Geometry check sheet. Reference: the model listing, model coordinates, mm. Coordinates: 2 decimals unless noted, no trailing zeros. Loops run counter-clockwise (first coordinate to the right, second up) from the corner with the lowest first, then second, coordinate; pieces in that order, holes last. Notation, with made-up numbers: (61.25, 71) -> (82.25, 71) arc R24 ccw to (82.25, 107) -> close; hole circle Ø8 at (39.5, -25.75). An arc over 180 degrees is marked (long way). Answer as a JSON object with one key per item and string values.
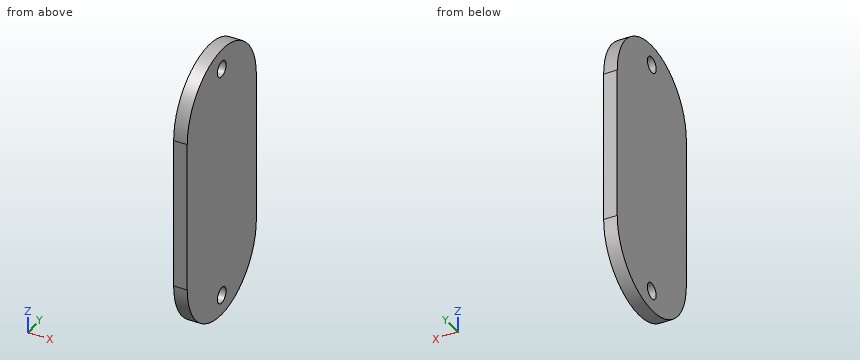
Autodesk Inventor part; units mm, degrees
ref_plane "YZ Plane" through (0, 0, 0) normal (1, 0, 0) x (0, 1, 0)
ref_plane "XZ Plane" through (0, 0, 0) normal (0, 1, 0) x (-1, 0, 0)
ref_plane "XY Plane" through (0, 0, 0) normal (0, 0, 1) x (1, 0, 0)
sketch "Sketch1" plane through (0, 0, 0) normal (1, 0, 0) x (0, 1, 0)
  arc A0 (-27.0381, 32.6694) -> (2.4619, 32.6694) centre (-12.2881, 32.6694) ccw
  arc A1 (-27.0381, 32.6694) -> (2.4619, 32.6694) centre (-12.2881, 32.6694) ccw
  arc A2 (-27.0381, 32.6694) -> (2.4619, 32.6694) centre (-12.2881, 32.6694) ccw
  line L0 (-27.0381, 32.6694) -> (-27.0381, 50.6694)
  line L1 (2.4619, 32.6694) -> (2.4619, 50.6694)
  line L2 (-27.0381, 50.6694) -> (-37.7302, 50.6694)
  arc A3 (2.4619, 68.6694) -> (-27.0381, 68.6694) centre (-12.2881, 68.6694) ccw
  arc A4 (2.4619, 68.6694) -> (-27.0381, 68.6694) centre (-12.2881, 68.6694) ccw
  arc A5 (2.4619, 68.6694) -> (-27.0381, 68.6694) centre (-12.2881, 68.6694) ccw
  line L3 (-27.0381, 68.6694) -> (-27.0381, 50.6694)
  line L4 (2.4619, 68.6694) -> (2.4619, 50.6694)
  circle A6 centre (-12.2881, 22.6694) radius 1.875
  circle A7 centre (-12.2881, 78.6694) radius 1.875
  point P0 (0, 0)
  dimension "d7" = 29.5
  dimension "d8" = 29.5
  dimension "d9" = 29.5
  dimension "d12" = 18
  dimension "d13" = 18
  dimension "d14" = 3.75
  dimension "d16" = 3.75
  dimension "d17" = 56
extrude "Extrusion1" add sketch "Sketch1" along normal blind 3.175
properties part number "clamp"
1. Section check B-B, the plane z = 22. Record the boundary of the cut face in (x, y) (3 decimals), then the cut area to 3 significant figures.
Evaluation:
{"outline": "(0, -22.473) -> (3.175, -22.473) -> (3.175, -14.04) -> (0, -14.04) -> close; (0, -10.537) -> (3.175, -10.537) -> (3.175, -2.103) -> (0, -2.103) -> close", "area": "53.6 mm^2"}
2. Section check D-D, the plane y = -24.25. Record the boundary of the cut face in (x, z) (3 decimals), then the cut area to 3 significant figures.
Evaluation:
{"outline": "(0, 24.039) -> (3.175, 24.039) -> (3.175, 77.299) -> (0, 77.299) -> close", "area": "169 mm^2"}
3. Thickness scan on probe 1 along Z at (x, y) = (0.5, -13.25); probe 2 along Y at (x, z) = (2.6, 80); probe 3 along Y at (x, z) = (2.7, 24). Record the ranges inside material, lowest first. Write a range as from..to.
Evaluation:
{"probe 1": "z = 17.95..21.06, 24.28..77.06, 80.28..83.39", "probe 2": "y = -21.73..-13.61, -10.97..-2.84", "probe 3": "y = -24.22..-13.61, -10.97..-0.35"}
4. Depth check by flat-ended pin: P1, Ø6, axis at y = -12.29, z = 22.67, coming from the +X side (3 decimals). Enter the tip coordinate at first touch or a pass-through.
Evaluation:
{"P1": "stops at x = 3.175"}
5. Section check A-A, the plane y = -11.5. Record the boundary of the cut face in (x, z) (3 decimals), then the cut area to 3 significant figures.
Evaluation:
{"outline": "(0, 17.94) -> (3.175, 17.94) -> (3.175, 20.968) -> (0, 20.968) -> close; (0, 24.371) -> (3.175, 24.371) -> (3.175, 76.968) -> (0, 76.968) -> close; (0, 80.371) -> (3.175, 80.371) -> (3.175, 83.398) -> (0, 83.398) -> close", "area": "186 mm^2"}
6. Section check C-C, the plane x = 1.15. Record the boundary of the cut face in (y, z) (3 decimals).
Evaluation:
{"outline": "(-27.038, 32.669) arc R14.75 ccw to (2.462, 32.669) -> (2.462, 68.669) arc R14.75 ccw to (-27.038, 68.669) -> close; hole circle Ø3.75 at (-12.288, 22.669); hole circle Ø3.75 at (-12.288, 78.669)"}
